```python
from build123d import *

# Parameters (mm, degrees)
SKETCH1_W           = 190
SKETCH1_H           = 190
BOSS_EXTRUDE1_DEPTH = 120
SKETCH2_W           = 120
SKETCH2_H           = 120
CUT_EXTRUDE1_DEPTH  = 117
SKETCH3_W           = 184
SKETCH3_H           = 184
SKETCH3_W_2         = 126
SKETCH3_H_2         = 126
CUT_EXTRUDE2_DEPTH  = 115
CUT_EXTRUDE3_DEPTH  = 53
SKETCH5_R           = 2.5
CUT_EXTRUDE4_DEPTH  = 17


with BuildPart() as part:
    # Sketch1 → Boss-Extrude1 (new body)
    with BuildSketch(Plane(origin=(0, 0, 0), x_dir=(1, 0, 0), z_dir=(0, 1, 0))):
        Rectangle(SKETCH1_W, SKETCH1_H)
    extrude(amount=BOSS_EXTRUDE1_DEPTH)

    # Sketch2 → Cut-Extrude1 (cut)
    with BuildSketch(Plane(origin=(0, 120, 0), x_dir=(1, 0, 0), z_dir=(0, 1, 0))):
        Rectangle(SKETCH2_W, SKETCH2_H)
    extrude(amount=-CUT_EXTRUDE1_DEPTH, mode=Mode.SUBTRACT)

    # Sketch3 → Cut-Extrude2 (cut)
    with BuildSketch(Plane(origin=(0, 120, 0), x_dir=(1, 0, 0), z_dir=(0, 1, 0))):
        Rectangle(SKETCH3_W, SKETCH3_H)
        Rectangle(SKETCH3_W_2, SKETCH3_H_2, mode=Mode.SUBTRACT)
    extrude(amount=-CUT_EXTRUDE2_DEPTH, mode=Mode.SUBTRACT)

    # Sketch4 → Cut-Extrude3 (cut)
    with BuildSketch(Plane(origin=(0, 5, 0), x_dir=(1, 0, 0), z_dir=(0, 1, 0))):
        Polygon((-89, -89), (-89, 89), (-63, 63), (-63, -63), align=None)
        Polygon((89, -89), (63, -63), (63, 63), (89, 89), align=None)
    extrude(amount=-CUT_EXTRUDE3_DEPTH, mode=Mode.SUBTRACT)

    # Sketch5 → Cut-Extrude4 (cut)
    with BuildSketch(Plane.XY.offset(63)):
        with Locations((0, 115)):
            Circle(SKETCH5_R)
    extrude(amount=-CUT_EXTRUDE4_DEPTH, mode=Mode.SUBTRACT)


solid = part.part
```
Here's how the part is built. I have some questions about the finished solid (model axes, mm). A direction names the side the tool comes from. Round coordinates to 2 decimals unless told otherwise and drop trailing zeros. Write each loop counter-clockwise with the first axis right and the second up, starting at its lowest first coordinate (ties: lowest second). Pieces come first, ordered by that corner, then holes. Notation, with made-up numbers: M 31,16 L 66,16 A13 cw 66,24 Z; hole C 11,58 d7. An arc over 180 degrees is marked long. Answer as CSV lines item,"result". Start each with the question number.
1. Suppose I cut it at C-C on x = 0. Write out the boundary of the cut face in (y, z).
2. Thinking about a two-plate mould opening in Z: for faces 4 (the flat face through (-1, 0, -1)), 5 (the flat face through (-1, 63, -92)), 6 (the flat face through (-1, 63, 63)), which applies, released by +Z, released by -Z, zero draft, split by the parting line, or undercut?
3. Suppose I cut it at B-B on z = 68.5. Write out the boundary of the cut face in (x, y).
4. I need wall thicknesses on probe 1 along Z at (x, y) = (-13, 106); probe 2 along Y at (x, z) = (0, 61.05). Which ranges of each line are inside material? Lowest first, please.
5. On a 3-axis mill with a long thin cutter (end or side, diameter ignored), from which of +Z, -Z, +X, -X, +Y, -Y can I reach the whole of each face in a straight line? I mean faces 1 (the flat face through (95, 59, 1)), 2 (the flat face through (76, 3, -76)), 3 (the flat face through (-92, 63, 1)). Say none if no direction works.
6. Suppose I cut it at D-D on z = -39. Write out the boundary of the cut face in (x, y).
7. I'm going to push a flat-ended pin straight in: pin 1 Ø5 at (x, z) = (-36, -71.5) entering from +Y. Where does the tip first touch, or does it pass through?
8. Suppose I cut it at A-A on y = 51.5. Write out the boundary of the cut face in (x, z), then the cut area to 3 significant figures.
Check result:
1,outline,"M 0,-95 L 120,-95 L 120,-92 L 5,-92 L 5,-63 L 120,-63 L 120,-60 L 3,-60 L 3,60 L 112.5,60 L 112.5,63 L 5,63 L 5,92 L 120,92 L 120,95 L 0,95 Z; M 117.5,60 L 120,60 L 120,63 L 117.5,63 Z"
2,face 4,"zero draft"
2,face 5,"undercut"
2,face 6,"undercut"
3,outline,"M -95,0 L -89,0 L -89,5 L -92,5 L -92,120 L -95,120 Z; M -68.5,0 L 68.5,0 L 68.5,5 L -68.5,5 Z; M 89,0 L 95,0 L 95,120 L 92,120 L 92,5 L 89,5 Z"
4,probe 1,"z = -95 to -92, -63 to -60, 60 to 63, 92 to 95"
4,probe 2,"y = 0 to 112.5, 117.5 to 120"
5,face 1,"+Z, -Z, +X, +Y, -Y"
5,face 2,"+Y, -Y"
5,face 3,"+Y"
6,outline,"M -95,0 L -89,0 L -89,5 L -92,5 L -92,120 L -95,120 Z; M -63,0 L 63,0 L 63,120 L 60,120 L 60,3 L -60,3 L -60,120 L -63,120 Z; M 89,0 L 95,0 L 95,120 L 92,120 L 92,5 L 89,5 Z"
7,pin 1,"stops at y = 5"
8,outline,"M -95,-95 L 95,-95 L 95,95 L -95,95 Z; M -63,-63 L 63,-63 L 63,63 L -63,63 Z; hole M -92,-92 L 92,-92 L 92,92 L -92,92 Z; hole M -60,-60 L 60,-60 L 60,60 L -60,60 Z"
8,area,"3,720 mm2"
